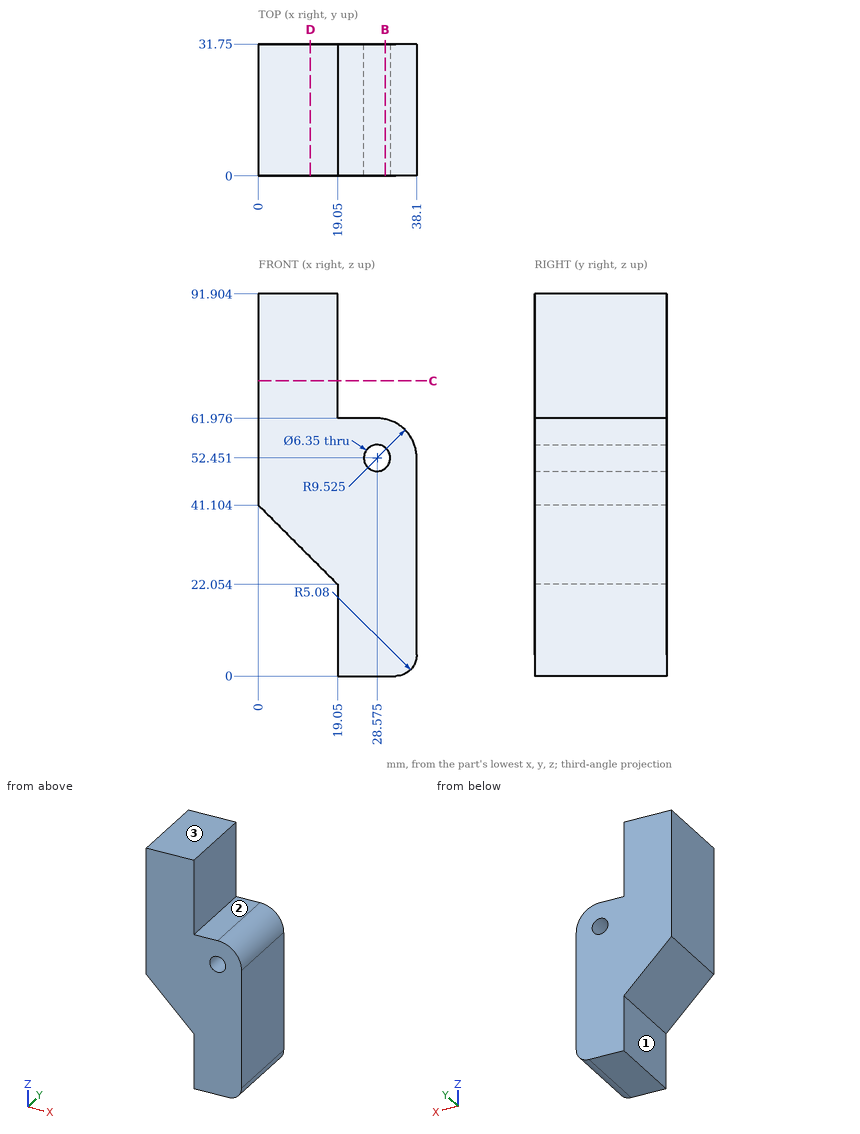
The figure shows three views and two pictorial views of one solid part (mm, origin at its lowest corner). Answer the questions. A direction names the side the tool comes from. Round coordinates to 2 decimals unless told otherwise and drop trailing zeros. Order: outer loops, then holes, each group sorted by start corner. A loop starts at its lowest first (then second) coordinate and runs counter-clockwise, first axis right, second up.
Q1. A cutting plane is placed at D-D, the plane x = 12.5. Determine the outline of the cut face in (y, z), then the cut area to 3 significant figures.
Solution:
outline: (0, 28.6) - (31.75, 28.6) - (31.75, 91.9) - (0, 91.9) - close
area: 2,010 mm2
Q2. A cutting plane is placed at C-C, the plane z = 71. Determine the outline of the cut face in (x, y).
Solution:
outline: (0, 0) - (19.05, 0) - (19.05, 31.75) - (0, 31.75) - close
Q3. A cutting plane is placed at B-B, the plane x = 30.5. Determine the outline of the cut face in (y, z), then the cut area to 3 significant figures.
Solution:
outline: (0, 0) - (31.75, 0) - (31.75, 49.93) - (0, 49.93) - close; (0, 54.98) - (31.75, 54.98) - (31.75, 61.78) - (0, 61.78) - close
area: 1,800 mm2
Q4. Given pin 1 Ø1.5 at (x, y) = (13.5, 5) entering from -Z (1 decimal); pin 2 Ø9 at (y, z) = (21, 79.5) entering from +X; pin 3 Ø10 at (x, y) = (31.5, 17.5) entering from +Z, each flat-ended and moving along its own axis, determine where each tip first touches the part or whether it passes through.
Solution:
pin 1: stops at z = 26.9
pin 2: stops at x = 19.05
pin 3: stops at z = 61.98
Q5. A tool of negligible diameter and unlimited length cuts with its end or side. For the marked faces 1, 2 and 3, from which of +Z, -Z, +X, -X, +Y, -Y can it reach the whole face along a straight path? Write none if from no direction.
Solution:
face 1: -Z, -X, +Y, -Y
face 2: +Z, +X, +Y, -Y
face 3: +Z, +X, -X, +Y, -Y
Q6. Find the intervals of material crossed by line 1 along X through (y, z) = (30.5, 85); line 2 along Z through (x, y) = (23.5, 8.5); line 3 along X through (y, z) = (22.5, 20), in increasing order.
Solution:
line 1: x = 0 to 19.05
line 2: z = 0 to 61.98
line 3: x = 19.05 to 38.1
